CAD build for the part. Positions are in the model's coordinates, mm. Coordinates: 2 decimals unless noted, no trailing zeros. Write each loop counter-clockwise with the first axis right and the second up, starting at its lowest first coordinate (ties: lowest second). Pieces come first, ordered by that corner, then holes.
```python
from build123d import *

# Parameters (mm, degrees)
SKETCH_1_R             = 6
SKETCH_1_R_2           = 5
EXTRUDE_1_DEPTH        = 200
SKETCH_4_R             = 1.6
CUT_EXTRUDE_2_DEPTH    = 201.179919073
PATTERN_LINEAR_1_COUNT = 6
PATTERN_LINEAR_1_PITCH = 15


with BuildPart() as part:
    # 草图1 → 凸台-拉伸1 (new body)
    with BuildSketch(Plane(origin=(0, 0, 0), x_dir=(1, 0, 0), z_dir=(0, 1, 0))):
        with Locations(Location((0, 0, 0), (0, 0, 270))):
            Circle(SKETCH_1_R)
        with Locations(Location((0, 0, 0), (0, 0, 270))):
            Circle(SKETCH_1_R_2, mode=Mode.SUBTRACT)
    extrude(amount=EXTRUDE_1_DEPTH)

    # 草图4 → 切除-拉伸2 (cut, symmetric)
    with BuildSketch(Plane(origin=(0, 0, 0), x_dir=(0, 0, -1), z_dir=(1, 0, 0))):
        with Locations((0, 15)):
            Circle(SKETCH_4_R)
    cut_extrude_2 = extrude(amount=CUT_EXTRUDE_2_DEPTH, both=True, mode=Mode.SUBTRACT)

    # 阵列(线性)1: 切除-拉伸2 ×6
    with Locations(*[(0, i * PATTERN_LINEAR_1_PITCH, 0) for i in range(1, PATTERN_LINEAR_1_COUNT)]):
        add(cut_extrude_2, mode=Mode.SUBTRACT)


solid = part.part
```
Item 1: Wall check: line 1 along X through (y, z) = (167.5, -0.5); line 2 along X through (y, z) = (83, -1.5); line 3 along Z through (x, y) = (5.4, 60). Give the ranges that are in metal, low to high.
Item 2: Two-plate mould, pull along Y, no slides. Class faces 1 (the flat face through (4, 200, -4)), 2 (the cylindrical face through (5.38, 43.58, -0.74)), 3 (the cylindrical face through (-5.857, 98.6, -1.301)): +Y half, -Y half, draft (parallel to the pull), parting line (faces both ways), or undercut.
Item 3: Flat gauge pins, fed straight in: pin 1 Ø5 at (y, z) = (15, 0) entering from +X; pin 2 Ø3 at (y, z) = (142.5, -4.5) entering from +X; pin 3 Ø4 at (y, z) = (101, 3) entering from +X; pin 4 Ø3 at (y, z) = (113.5, 2) entering from -X. Where does each tip first touch, or does it go through?
Item 4: Saw through at B-B, the plane y = 123.5. Write the cut outline in (x, z).
Item 5: Saw through at A-A, the plane x = 2. Write the cut outline in (y, z).
Working result:
1. line 1: x = -5.98 to -4.97, 4.97 to 5.98
1. line 2: x = -5.81 to -4.77, 4.77 to 5.81
1. line 3: z = -2.62 to -1.6, 1.6 to 2.62
2. face 1: +Y half
2. face 2: undercut
2. face 3: draft
3. pin 1: stops at x = 6
3. pin 2: stops at x = 5.2
3. pin 3: stops at x = 5.92
3. pin 4: stops at x = -5.98
4. outline: circle Ø12 at (0, 0); hole circle Ø10 at (0, 0)
5. outline: (0, -5.66) - (200, -5.66) - (200, -4.58) - (0, -4.58) - close; (0, 4.58) - (200, 4.58) - (200, 5.66) - (0, 5.66) - close
